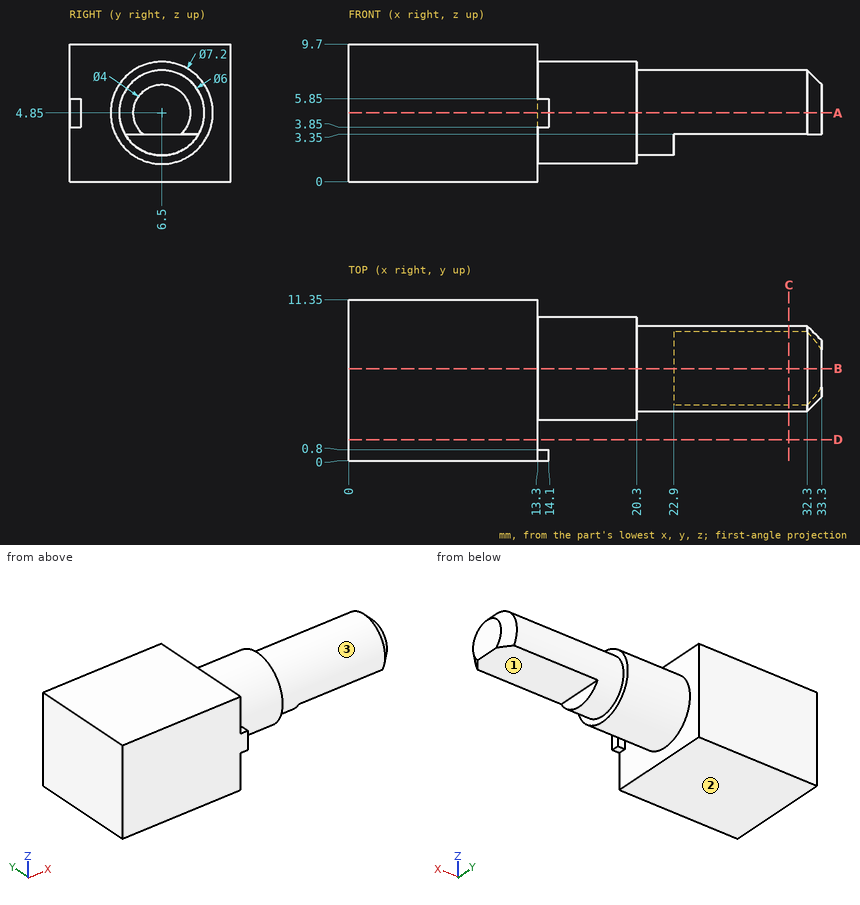
Input: dimensioned drawing with shaded views. Units: mm. Origin: part minimum x, y, z. A direction names the side the tool comes from. Coordinates: 2 decimals unless noted, no trailing zeros. Order: outer loops, then holes, each group sorted by start corner. A loop starts at its lowest first (then second) coordinate and runs counter-clockwise, first axis right, second up. Notation, with made-up numbers: (86, 23.5) - (95, 23.5) arc R24 ccw to (95, 59.5) - close; hole circle Ø6 at (50.5, 50.5). An arc over 180 degrees is marked (long way). Return JSON: item names as keys, results as strings. Group by question number.
1. Cut plane D-D (y = 1.5). Output: boundary loops of the cut face in (x, z).
2. Cut plane C-C (x = 31). Output: boundary loops of the cut face in (y, z), plus the area to 3 significant figures.
3. Material intervals for line 1 along X through (y, z) = (5.5, 1.25); line 2 along X through (y, z) = (0.5, 5.5); line 3 along Z through (x, y) = (27.5, 7), sorted ascending. Write a range as [from, to].
4. Set-up query: the marked faces 1, 2 and 3. Return all of +Z, -Z, +X, -X, +Y, -Y with unobstructed straight access to the full face (end or side cutting, diameter ignored); none if empty.
5. Cut plane B-B (y = 6.5). Output: boundary loops of the cut face in (x, z).
6. Cut plane A-A (z = 4.85). Output: boundary loops of the cut face in (x, y), plus the area to 3 significant figures.
7. Pin query (flat end, axial travel): pin 1 (4 mm diameter, centred on x = 20.5, y = 5.5, fed in from -Z); pin 2 (0.6 mm diameter, centred on y = 0.5, z = 4.5, fed in from +X); pin 3 (4 mm diameter, centred on x = 28.5, z = 6, fed in from +Y). Return the tip coordinate at first contact, or that it passes through.
Resolved:
{
 "1": {"outline": "(0, 0) - (13.3, 0) - (13.3, 9.7) - (0, 9.7) - close"},
 "2": {"outline": "(3.9, 3.35) - (9.1, 3.35) arc R3 ccw (long way) to start", "area": "22.7 mm²"},
 "3": {"line 1": "x = [0, 13.3]", "line 2": "x = [0, 14.1]", "line 3": "z = [3.35, 7.81]"},
 "4": {"face 1": "-Z, +X, +Y, -Y", "face 2": "-Z, +X, -X, +Y, -Y", "face 3": "+X"},
 "5": {"outline": "(0, 0) - (13.3, 0) - (13.3, 1.25) - (20.3, 1.25) - (20.3, 1.85) - (22.9, 1.85) - (22.9, 3.35) - (33.3, 3.35) - (33.3, 6.85) - (32.3, 7.85) - (20.3, 7.85) - (20.3, 8.45) - (13.3, 8.45) - (13.3, 9.7) - (0, 9.7) - close"},
 "6": {"outline": "(0, 0) - (14.1, 0) - (14.1, 0.8) - (13.3, 0.8) - (13.3, 2.9) - (20.3, 2.9) - (20.3, 3.5) - (32.3, 3.5) - (33.3, 4.5) - (33.3, 8.5) - (32.3, 9.5) - (20.3, 9.5) - (20.3, 10.1) - (13.3, 10.1) - (13.3, 11.35) - (0, 11.35) - close", "area": "279 mm²"},
 "7": {"pin 1": "stops at z = 1.25", "pin 2": "stops at x = 14.1", "pin 3": "stops at y = 9.5"}
}
